Verification items for the finished model (mm, model axes). Face numbers are marked on the shaded views. A direction names the side the tool comes from. Coordinates: 2 decimals unless noted, no trailing zeros. Loops run counter-clockwise (first coordinate to the right, second up) from the corner with the lowest first, then second, coordinate; pieces in that order, holes last. Notation, with made-up numbers: M -32.75,15.5 L -0.75,15.5 A11 cw -0.75,27.5 Z; hole C 60.25,16 d7. An arc over 180 degrees is marked long. Write item = value, one per line. Start each with the question number.
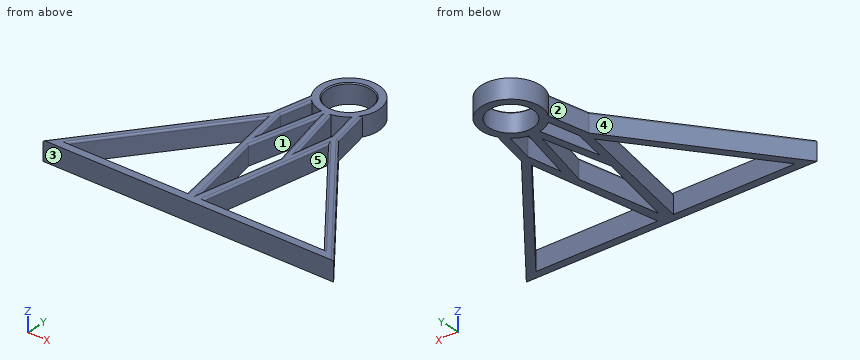
```python
from build123d import *

# Parameters (mm, degrees)
F0_R     = 11.25
F1_DEPTH = 10
F2_DEPTH = 7.1
F3_R     = 1
F5_SIZE  = 0.5


# Not quite as in the source:
# - two fillets or chamfers of one size are made in one step
# - a feature names something its author has since deleted; it is built from what else it names


with BuildPart() as f1:
    # F0 (on Top) → F1 (new body)
    with BuildSketch(Plane.XY):
        with BuildLine():
            ThreePointArc((-2.8618452925, -14.9790634394), (0, -15.25), (2.8618452925, -14.9790634394))
            ThreePointArc((2.8618452925, -14.9790634394), (6.5768557716, -13.7589050494), (9.8594632948, -11.6341516037))
            ThreePointArc((9.8594632948, -11.6341516037), (11.6573360398, -9.8320402997), (13.1303972918, -7.7559762093))
            ThreePointArc((13.1303972918, -7.7559762093), (0, 15.25), (-13.1303972918, -7.7559762093))
            ThreePointArc((-13.1303972918, -7.7559762093), (-11.6573360398, -9.8320402997), (-9.8594632948, -11.6341516037))
            ThreePointArc((-9.8594632948, -11.6341516037), (-6.5768557716, -13.7589050494), (-2.8618452925, -14.9790634394))
        make_face()
        Circle(F0_R, mode=Mode.SUBTRACT)
        with BuildLine():
            Line((10.0593915347, -44.4443559719), (2.8618452925, -14.9790634394))
            ThreePointArc((2.8618452925, -14.9790634394), (0, -15.25), (-2.8618452925, -14.9790634394))
            Line((-2.8618452925, -14.9790634394), (-10.0593915347, -44.4443559719))
            Line((-10.0593915347, -44.4443559719), (-13.1918562915, -27.455889859))
            Line((-13.1918562915, -27.455889859), (-9.8594632948, -11.6341516037))
            ThreePointArc((-9.8594632948, -11.6341516037), (-11.6573360398, -9.8320402997), (-13.1303972918, -7.7559762093))
            Line((-13.1303972918, -7.7559762093), (-17.4770367352, -28.3932154638))
            Line((-17.4770367352, -28.3932154638), (-75, -103))
            Line((-75, -103), (75, -103))
            Line((75, -103), (17.4770367352, -28.3932154638))
            Line((17.4770367352, -28.3932154638), (13.1303972918, -7.7559762093))
            ThreePointArc((13.1303972918, -7.7559762093), (11.6573360398, -9.8320402997), (9.8594632948, -11.6341516037))
            Line((9.8594632948, -11.6341516037), (13.1918562915, -27.455889859))
            Line((13.1918562915, -27.455889859), (10.0593915347, -44.4443559719))
        make_face()
        Polygon((-66.8650551594, -99), (-16.187040587, -33.2710545609), (-4.0674293329, -99), align=None, mode=Mode.SUBTRACT)
        Polygon((66.8650551594, -99), (4.0674293329, -99), (16.187040587, -33.2710545609), align=None, mode=Mode.SUBTRACT)
        Polygon((-8.2882046257, -54.0501300567), (0, -20.1199036092), (8.2882046257, -54.0501300567), (0, -94.5818126202), align=None, mode=Mode.SUBTRACT)
    extrude(amount=F1_DEPTH)

    # F0 (on Top) → F2 (join)
    with BuildSketch(Plane.XY):
        with BuildLine():
            ThreePointArc((-2.8618452925, -14.9790634394), (0, -15.25), (2.8618452925, -14.9790634394))
            ThreePointArc((2.8618452925, -14.9790634394), (6.5768557716, -13.7589050494), (9.8594632948, -11.6341516037))
            ThreePointArc((9.8594632948, -11.6341516037), (11.6573360398, -9.8320402997), (13.1303972918, -7.7559762093))
            ThreePointArc((13.1303972918, -7.7559762093), (0, 15.25), (-13.1303972918, -7.7559762093))
            ThreePointArc((-13.1303972918, -7.7559762093), (-11.6573360398, -9.8320402997), (-9.8594632948, -11.6341516037))
            ThreePointArc((-9.8594632948, -11.6341516037), (-6.5768557716, -13.7589050494), (-2.8618452925, -14.9790634394))
        make_face()
        Circle(F0_R, mode=Mode.SUBTRACT)
    extrude(amount=F2_DEPTH)

    # F3
    f3_edges = [f1.edges().sort_by_distance(p)[0] for p in [
        (-15.303717, -18.074596, 10),
        (-11.52566, -19.545021, 10),
        (-11.625624, -35.950123, 10),
        (-46.238518, -65.696608, 10),
        (-41.526048, -66.135527, 10),
        (-10.127235, -66.135527, 10),
        (-6.460618, -29.71171, 10),
        (6.460618, -29.71171, 10),
        (11.52566, -19.545021, 10),
        (11.625624, -35.950123, 10),
        (15.303717, -18.074596, 10),
        (46.238518, -65.696608, 10),
        (41.526048, -66.135527, 10),
        (10.127235, -66.135527, 10),
        (-4.144102, -37.085017, 10),
        (-4.144102, -74.315971, 10),
        (4.144102, -74.315971, 10),
        (4.144102, -37.085017, 10),
    ]]
    fillet(f3_edges, radius=F3_R)

    # F5
    f5_edges = [f1.edges().sort_by_distance(p)[0] for p in [
        (-11.25, 0, 10),
    ]]
    chamfer(f5_edges, length=F5_SIZE)


solid = f1.part
```
Q1. Mould release check, pull along Y, two halves, no side actions. Record for the marked faces 3, 4 and 5: +Y half, -Y half, draft (parallel to the pull), parting line (faces both ways), or undercut.
Q2. Gauge pin test, flat ends, axial feed: pin 1 (20 mm diameter, centred on x = 0, y = 0, fed in from +Z); pin 2 (3 mm diameter, centred on x = 28, z = 6.5, fed in from +Y); pin 3 (5 mm diameter, centred on y = -64, z = 7, fed in from -X); pin 4 (1 mm diameter, centred on y = -60.5, z = 3, fed in from -X). Record the tip position at first contact, or that the pin passes through.
Q3. Scan lines: L1, parallel to X at y = -90.5, z = 7.25; L2, parallel to X at y = -52.5, z = 5.5; L3, parallel to X at y = -12.5, z = 8.25. Record each from-to range of solid material in increasing order. Write a range as [from, to].
Q4. Sectioned sample at B-B on z = 3.25. Record the cut outline in (x, y).
Q5. Sectioned sample at C-C on y = -58. Count the separate pieces of the cut face and the enclosed holes in it, plus the area to 3 significant figures.
Q6. Sectioned sample at A-A on y = 0. Record the cut outline in (x, z).
Q7. Set-up check for the marked faces 1 and 2: record each of +Z, -Z, +X, -X, +Y, -Y from which the full face is reachable in a straight line by a thin tool's end or side.
Solutions:
q1.face_3 = -Y half
q1.face_4 = +Y half
q1.face_5 = undercut
q2.pin_1 = through
q2.pin_2 = -40.1
q2.pin_3 = -46.86
q2.pin_4 = -42.62
q3.L1 = [-65.36, -60.31], [-5.63, -0.83], [0.83, 5.63], [60.31, 65.36]
q3.L2 = [-36.06, -31.01], [-12.64, -7.91], [7.91, 12.64], [31.01, 36.06]
q3.L3 = [-14.13, -10.04], [-8.74, 8.74], [10.04, 14.13]
q4.outline = M -75,-103 L 75,-103 L 17.48,-28.39 L 13.13,-7.76 A15.25 ccw long -13.13,-7.76 L -17.48,-28.39 Z; hole M -66.87,-99 L -4.07,-99 L -16.19,-33.27 Z; hole M -13.19,-27.46 L -10.06,-44.44 L -2.86,-14.98 A15.25 cw -9.86,-11.63 Z; hole C 0,0 d22.5; hole M -8.29,-54.05 L 0,-94.58 L 8.29,-54.05 L 0,-20.12 Z; hole M 2.86,-14.98 L 10.06,-44.44 L 13.19,-27.46 L 9.86,-11.63 A15.25 cw Z; hole M 4.07,-99 L 66.87,-99 L 16.19,-33.27 Z
q5.separate_pieces = 4
q5.enclosed_holes = 0
q5.area = 182 mm²
q6.outline = M -15.25,0 L -11.25,0 L -11.25,9.5 L -11.75,10 L -15.25,10 Z; M 11.25,0 L 15.25,0 L 15.25,10 L 11.75,10 L 11.25,9.5 Z
q7.face_1 = +Z, -Z
q7.face_2 = +Z, -Z, -X
